```python
from build123d import *

# Parameters (mm, degrees)
CROQUIS2_R              = 2.5
SALIENTE_EXTRUIR1_DEPTH = 8
CROQUIS3_R              = 3.5
CORTAR_EXTRUIR1_DEPTH   = 1
CROQUIS4_R              = 3.5
CORTAR_EXTRUIR2_DEPTH   = 1


with BuildPart() as part:
    # Croquis2 → Saliente-Extruir1 (new body)
    with BuildSketch(Plane(origin=(0, 0, 0), x_dir=(1, 0, 0), z_dir=(0, 1, 0))):
        with BuildLine():
            Line((-6.5, 70), (-6.5, 0))
            ThreePointArc((-6.5, 0), (0, -6.5), (6.5, 0))
            Line((6.5, 0), (6.5, 24))
            ThreePointArc((6.5, 24), (9.428932188, 31.071067812), (16.5, 34))
            Line((16.5, 34), (19.5, 34))
            Line((19.5, 34), (21.621320344, 36.121320344))
            Line((21.621320344, 36.121320344), (19.621320344, 38.121320344))
            Line((19.621320344, 38.121320344), (21.621320344, 40.121320344))
            Line((21.621320344, 40.121320344), (19.621320344, 42.121320344))
            Line((19.621320344, 42.121320344), (21.621320344, 44.121320344))
            ThreePointArc((21.621320344, 44.121320344), (8.897927721, 59.859277281), (13.535653981, 79.558503244))
            Line((13.535653981, 79.558503244), (11.21874212, 81.180822395))
            Line((11.21874212, 81.180822395), (12.841061271, 83.497734256))
            Line((12.841061271, 83.497734256), (10.524149409, 85.120053407))
            Line((10.524149409, 85.120053407), (12.14646856, 87.436965268))
            Line((12.14646856, 87.436965268), (9.829556699, 89.059284419))
            Line((9.829556699, 89.059284419), (11.451875849, 91.37619628))
            Line((11.451875849, 91.37619628), (11.174038765, 92.951888685))
            Line((11.174038765, 92.951888685), (6.25, 92.083647797))
            Line((6.25, 92.083647797), (-6.5, 70))
        make_face()
        Circle(CROQUIS2_R, mode=Mode.SUBTRACT)
        with Locations((0, 30)):
            Circle(CROQUIS2_R, mode=Mode.SUBTRACT)
    extrude(amount=SALIENTE_EXTRUIR1_DEPTH)

    # Croquis3 → Cortar-Extruir1 (cut)
    with BuildSketch(Plane(origin=(0, 8, 0), x_dir=(1, 0, 0), z_dir=(0, 1, 0))):
        with BuildLine():
            Line((7.515743149, 90.275979241), (-4.5, 69.464101615))
            Line((-4.5, 69.464101615), (6.386283079, 63.178903149))
            ThreePointArc((6.386283079, 63.178903149), (7.166644063, 71.420557609), (10.59569924, 78.955503667))
            Line((10.59569924, 78.955503667), (8.566911861, 90.461328646))
            Line((8.566911861, 90.461328646), (7.515743149, 90.275979241))
        make_face()
        with BuildLine():
            Line((-4.5, 67.154700538), (-4.5, 43.774315056))
            Line((-4.5, 43.774315056), (14.183644035, 43.774315056))
            Line((14.183644035, 43.774315056), (14.183644035, 46.774315056))
            ThreePointArc((14.183644035, 46.774315056), (9.308263877, 53.126130169), (6.691099089, 60.693516467))
            Line((6.691099089, 60.693516467), (-4.5, 67.154700538))
        make_face()
        with BuildLine():
            Line((-4.5, 2.828427125), (-4.5, 41.774315056))
            Line((-4.5, 41.774315056), (14.183644035, 41.774315056))
            Line((14.183644035, 41.774315056), (14.183644035, 35.774315056))
            ThreePointArc((14.183644035, 35.774315056), (7.231875282, 31.622457885), (4.5, 24))
            Line((4.5, 24), (4.5, 2.828427125))
            Line((4.5, 2.828427125), (3.5, 2.828427125))
            ThreePointArc((3.5, 2.828427125), (0, 4.5), (-3.5, 2.828427125))
            Line((-3.5, 2.828427125), (-4.5, 2.828427125))
        make_face()
        with Locations((0, 30)):
            Circle(CROQUIS3_R, mode=Mode.SUBTRACT)
    extrude(amount=-CORTAR_EXTRUIR1_DEPTH, mode=Mode.SUBTRACT)

    # Croquis4 → Cortar-Extruir2 (cut)
    with BuildSketch(Plane.XZ):
        with BuildLine():
            Line((4.5, -24), (4.5, -2.828427125))
            Line((4.5, -2.828427125), (3.5, -2.828427125))
            ThreePointArc((3.5, -2.828427125), (0, -4.5), (-3.5, -2.828427125))
            Line((-3.5, -2.828427125), (-4.5, -2.828427125))
            Line((-4.5, -2.828427125), (-4.5, -41.774315056))
            Line((-4.5, -41.774315056), (14.183644035, -41.774315056))
            Line((14.183644035, -41.774315056), (14.183644035, -35.774315056))
            ThreePointArc((14.183644035, -35.774315056), (7.231875282, -31.622457885), (4.5, -24))
        make_face()
        with Locations((0, -30)):
            Circle(CROQUIS4_R, mode=Mode.SUBTRACT)
        with BuildLine():
            Line((6.386283079, -63.178903149), (-4.5, -69.464101615))
            Line((-4.5, -69.464101615), (7.515743149, -90.275979241))
            Line((7.515743149, -90.275979241), (8.566911861, -90.461328646))
            Line((8.566911861, -90.461328646), (10.59569924, -78.955503667))
            ThreePointArc((10.59569924, -78.955503667), (7.166644063, -71.420557609), (6.386283079, -63.178903149))
        make_face()
        with BuildLine():
            Line((-4.5, -67.154700538), (6.691099089, -60.693516467))
            ThreePointArc((6.691099089, -60.693516467), (9.308263877, -53.126130169), (14.183644035, -46.774315056))
            Line((14.183644035, -46.774315056), (14.183644035, -43.774315056))
            Line((14.183644035, -43.774315056), (-4.5, -43.774315056))
            Line((-4.5, -43.774315056), (-4.5, -67.154700538))
        make_face()
    extrude(amount=-CORTAR_EXTRUIR2_DEPTH, mode=Mode.SUBTRACT)


solid = part.part
```
Model file for the job. Use its own axes, mm. A direction names the side the tool comes from. Give positions to 0.01 mm unless a question says otherwise; leave off trailing zeros. Write each loop counter-clockwise with the first axis right and the second up, starting at its lowest first coordinate (ties: lowest second). Pieces come first, ordered by that corner, then holes. Notation, with made-up numbers: M 27.5,30 L 52.5,30 A15 cw 52.5,50 Z; hole C 81.25,71.25 d8. An arc over 180 degrees is marked long. Use a Markdown table: item, result.
1) Pull direction X, two halves, no side cores. Call faces 6 (the flat face through (-6.5, 4, -35)), 7 (the cylindrical face through (-0.46, 0.49, -26.53)), 8 (the flat face through (2, 0, -28)): +X half, -X half, draft (parallel to the pull), parting line (faces both ways), or undercut.
Responses:
| item | result |
|---|---|
| face 6 | -X half |
| face 7 | undercut |
| face 8 | draft |
2) Cut at C-C (z = -30). List the corners of the cut face in (x, y).
Responses:
| item | result |
|---|---|
| outline | M -6.5,0 L -4.5,0 L -4.5,1 L -3.5,1 L -3.5,0 L -2.5,0 L -2.5,8 L -3.5,8 L -3.5,7 L -4.5,7 L -4.5,8 L -6.5,8 Z; M 2.5,0 L 3.5,0 L 3.5,1 L 6.11,1 L 6.11,0 L 8.5,0 L 8.5,8 L 6.11,8 L 6.11,7 L 3.5,7 L 3.5,8 L 2.5,8 Z |
3) Drill centre lines: line 1 (Z direction, x = 0, y = 6.75); line 2 (Y direction, x = 3.5, z = -33.5); line 3 (X direction, y = 6.25, z = -3). Where is each one in solid material? Low to high. Write a range as from..to.
Responses:
| item | result |
|---|---|
| line 1 | z = -81.26..-32.5, -27.5..-2.5, 2.5..6.5 |
| line 2 | y = 1..7 |
| line 3 | x = -6.5..6.5 |
4) Cut at A-A (y = 3.5). List the corners of the cut face in (x, z).
Responses:
| item | result |
|---|---|
| outline | M -6.5,-70 L 6.25,-92.08 L 11.17,-92.95 L 11.45,-91.38 L 9.83,-89.06 L 12.15,-87.44 L 10.52,-85.12 L 12.84,-83.5 L 11.22,-81.18 L 13.54,-79.56 A23 cw 21.62,-44.12 L 19.62,-42.12 L 21.62,-40.12 L 19.62,-38.12 L 21.62,-36.12 L 19.5,-34 L 16.5,-34 A10 cw 6.5,-24 L 6.5,0 A6.5 ccw -6.5,0 Z; hole C 0,-30 d5; hole C 0,0 d5 |
5) Cut at B-B (z = -19.5). List the corners of the cut face in (x, y), and give its area (3 significant figures).
Responses:
| item | result |
|---|---|
| outline | M -6.5,0 L -4.5,0 L -4.5,1 L 4.5,1 L 4.5,0 L 6.5,0 L 6.5,8 L 4.5,8 L 4.5,7 L -4.5,7 L -4.5,8 L -6.5,8 Z |
| area | 86.0 mm2 |
6) Pin check, flat tips, straight feed: pin 1 (0.8 mm diameter, centred on x = -4, y = 7.5, fed in from -Z); pin 2 (2 mm diameter, centred on x = 18, y = 7, fed in from +Z); pin 3 (1 mm diameter, centred on y = 3.5, z = -12.5, fed in from +X). Stop position of each tip, or through.
Responses:
| item | result |
|---|---|
| pin 1 | stops at z = -75.02 |
| pin 2 | stops at z = -34 |
| pin 3 | stops at x = 6.5 |
7) Cut at D-D (x = 0). Give the number of separate pieces and of enclosed holes in the cut face, and give its area (3 significant figures).
Responses:
| item | result |
|---|---|
| separate pieces | 3 |
| enclosed holes | 0 |
| area | 499 mm2 |
8) Tool access for faces 1 (the flat face through (5, 0, -43)), 2 (the flat face through (0.867, 7.507, -66.365)), 3 (the flat face through (5, 1, -74)), 4 (the flat face through (12, 3.9, -82.3)), 5 (the flat face through (6.5, 4, -12)): list every direction of +Z, -Z, +X, -X, +Y, -Y with a clear straight run to the whole face (end or side of a thin tool).
Responses:
| item | result |
|---|---|
| face 1 | +Z, -Z, +X, -X, -Y |
| face 2 | +Y |
| face 3 | -Y |
| face 4 | +X, +Y, -Y |
| face 5 | +Z, +X, +Y, -Y |
